Geometry: final body of the model. Coordinates: model frame, mm. A direction names the side the tool comes from. Coordinates: 2 decimals unless noted, no trailing zeros. Write each loop counter-clockwise with the first axis right and the second up, starting at its lowest first coordinate (ties: lowest second). Pieces come first, ordered by that corner, then holes. Notation, with made-up numbers: M -40,-3 L 0,-3 A22 cw 0,12 Z; hole C 85.5,69 d4. An arc over 180 degrees is marked long. Write item = value, one per line. Start each with the question number.
Item 1: Reachability of faces 4 (the flat face through (6, 0, 32)), 5 (the flat face through (10, -15, -49)), 6 (the flat face through (-17.5, 5, 50)) from +Z, -Z, +X, -X, +Y, -Y: full face, straight path, thin tool, end or side. Return the list, or none.
Item 2: Section A-A on x = 0. Output: boundary loops of the cut face in (y, z).
Item 3: Ray query, L1, parallel to X at y = 1, z = 40.5; L2, parallel to X at y = -11.25, z = -50; L3, parallel to Y at x = -26.5, z = -22. Return the intervals inside material, ascending. Write a range as [from, to].
Item 4: Section B-B on z = 48. Output: boundary loops of the cut face in (x, y), plus the area to 3 significant figures.
Item 5: Section D-D on z = 0. Output: boundary loops of the cut face in (x, y), plus the area to 3 significant figures.
Item 6: First-contact query: pin 1 Ø7.5 at (x, z) = (-18.12, -32.26) entering from -Y; pin 2 Ø9 at (x, z) = (18.12, 32.26) entering from +Y; pin 3 Ø6 at (x, z) = (-2.5, -52) entering from -Y. Flat tips, straight axial feed; report the tip coordinate or a pass-through.
Item 7: Section C-C on y = -15.5. Output: boundary loops of the cut face in (x, z), plus the area to 3 significant figures.
Item 8: Pull-direction query (X, two-part tool) for faces 1 (the flat face through (17.5, 5, 50)), 2 (the flat face through (-2, -5, -60)), 3 (the flat face through (110, -5, -1)); classes: +X half, -X half, draft (parallel to the pull), parting line (faces both ways), or undercut.
from build123d import *

# Parameters (mm, degrees)
SKETCH1_W               = 220
SKETCH1_H               = 120
SKETCH1_R               = 43
BOSS_EXTRUDE1_DEPTH     = 10
SKETCH2_W               = 220
SKETCH2_H               = 120
SKETCH2_R               = 2.8
BOSS_EXTRUDE2_DEPTH     = 20
CUT_EXTRUDE1_REACH      = 166.012
CUT_EXTRUDE1_END_RADIUS = 43
SKETCH3_W               = 35
SKETCH3_H               = 10
SKETCH4_R               = 32
CUT_EXTRUDE2_DEPTH      = 127.885775404
CUT_EXTRUDE3_REACH      = 166.012
CUT_EXTRUDE3_END_RADIUS = 32
SKETCH5_W               = 20
SKETCH5_H               = 10
SKETCH6_R               = 42.5
CUT_EXTRUDE4_DEPTH      = 7


with BuildPart() as part:
    # Sketch1 → Boss-Extrude1 (new body)
    with BuildSketch(Plane(origin=(0, 0, 0), x_dir=(1, 0, 0), z_dir=(0, 1, 0))):
        Rectangle(SKETCH1_W, SKETCH1_H)
        with Locations(Location((0, 0, 0), (0, 0, 270))):
            Circle(SKETCH1_R, mode=Mode.SUBTRACT)
    extrude(amount=BOSS_EXTRUDE1_DEPTH)

    # Sketch2 → Boss-Extrude2 (add)
    with BuildSketch(Plane.XZ):
        Rectangle(SKETCH2_W, SKETCH2_H)
        with Locations(Location((18.122136771, 32.25814872, 0), (0, 0, 270))):
            Circle(SKETCH2_R, mode=Mode.SUBTRACT)
        with Locations(Location((36.997444656, 0.434843546, 0), (0, 0, 270))):
            Circle(SKETCH2_R, mode=Mode.SUBTRACT)
        with Locations(Location((18.875307886, -31.823305174, 0), (0, 0, 270))):
            Circle(SKETCH2_R, mode=Mode.SUBTRACT)
        with Locations(Location((-18.122136771, -32.25814872, 0), (0, 0, 270))):
            Circle(SKETCH2_R, mode=Mode.SUBTRACT)
        with Locations(Location((-36.997444656, -0.434843546, 0), (0, 0, 270))):
            Circle(SKETCH2_R, mode=Mode.SUBTRACT)
        with Locations(Location((-18.875307886, 31.823305174, 0), (0, 0, 270))):
            Circle(SKETCH2_R, mode=Mode.SUBTRACT)
    extrude(amount=BOSS_EXTRUDE2_DEPTH)

    # Cut-Extrude1: up to this cylinder (the profile starts outside it)
    cut_extrude1_end = Plane(origin=(0, 5, 0), z_dir=(0, -1, 0)) * Cylinder(CUT_EXTRUDE1_END_RADIUS, 419.024, mode=Mode.PRIVATE)
    # Sketch3 → Cut-Extrude1 (cut, up to the surface)
    with BuildSketch(Plane.XY.offset(60), mode=Mode.PRIVATE) as cut_extrude1_sk1:
        with Locations((0, 5)):
            Rectangle(SKETCH3_W, SKETCH3_H)
    cut_extrude1_tool1 = extrude(cut_extrude1_sk1.sketch, amount=-CUT_EXTRUDE1_REACH, mode=Mode.PRIVATE) - cut_extrude1_end
    add(cut_extrude1_tool1.solids().sort_by_distance((0, 5, 60))[0], mode=Mode.SUBTRACT)

    # Sketch4 → Cut-Extrude2 (cut, through all)
    with BuildSketch(Plane(origin=(0, 0, 0), x_dir=(1, 0, 0), z_dir=(0, 1, 0))):
        with Locations(Location((0, 0, 0), (0, 0, 270))):
            Circle(SKETCH4_R)
    extrude(amount=-CUT_EXTRUDE2_DEPTH, mode=Mode.SUBTRACT)

    # Cut-Extrude3: up to this cylinder (the profile starts outside it)
    cut_extrude3_end = Plane(origin=(0, -15, 0), z_dir=(0, 1, 0)) * Cylinder(CUT_EXTRUDE3_END_RADIUS, 397.024, mode=Mode.PRIVATE)
    # Sketch5 → Cut-Extrude3 (cut, up to the surface)
    with BuildSketch(Plane(origin=(0, 0, -60), x_dir=(-1, 0, 0), z_dir=(0, 0, -1)), mode=Mode.PRIVATE) as cut_extrude3_sk1:
        with Locations((0, -15)):
            Rectangle(SKETCH5_W, SKETCH5_H)
    cut_extrude3_tool1 = extrude(cut_extrude3_sk1.sketch, amount=-CUT_EXTRUDE3_REACH, mode=Mode.PRIVATE) - cut_extrude3_end
    add(cut_extrude3_tool1.solids().sort_by_distance((0, -15, -60))[0], mode=Mode.SUBTRACT)

    # Sketch6 → Cut-Extrude4 (cut)
    with BuildSketch(Plane.XZ.offset(20)):
        Circle(SKETCH6_R)
    extrude(amount=-CUT_EXTRUDE4_DEPTH, mode=Mode.SUBTRACT)


solid = part.part
Responses:
q1.face_4 = +Y
q1.face_5 = -Z, -Y
q1.face_6 = +Z, +Y
q2.outline = M -20,42.5 L -13,42.5 L -13,32 L 0,32 L 0,60 L -20,60 Z; M -10,-60 L 10,-60 L 10,-43 L 0,-43 L 0,-32 L -10,-32 Z
q3.L1 = [-110, -17.5], [17.5, 110]
q3.L2 = [-110, -10], [10, 110]
q3.L3 = [-13, 0]
q4.outline = M -110,-20 L 110,-20 L 110,10 L 17.5,10 L 17.5,0 L -17.5,0 L -17.5,10 L -110,10 Z
q4.area = 6,250 mm²
q5.outline = M -110,-20 L -42.5,-20 L -42.5,-13 L -39.76,-13 L -39.76,0 L -43,0 L -43,10 L -110,10 Z; M -34.23,-13 L -32,-13 L -32,0 L -34.23,0 Z; M 32,-13 L 34.23,-13 L 34.23,0 L 32,0 Z; M 39.76,-13 L 42.5,-13 L 42.5,-20 L 110,-20 L 110,10 L 43,10 L 43,0 L 39.76,0 Z
q5.area = 4,170 mm²
q6.pin_1 = -13
q6.pin_2 = 0
q6.pin_3 = -10
q7.outline = M -110,-60 L -10,-60 L -10,-41.31 A42.5 cw long 10,-41.31 L 10,-60 L 110,-60 L 110,60 L -110,60 Z
q7.area = 20,400 mm²
q8.face_1 = undercut
q8.face_2 = draft
q8.face_3 = +X half
